```python
from build123d import *

# Parameters (mm, degrees)
SKETCH_1_W             = 60
SKETCH_1_H             = 30
EXTRUDE_1_DEPTH        = 8
CUT_EXTRUDE_1_REACH    = 10
SKETCH_2_R             = 1.2
HOLE_WIZARD_M3_1_D     = 2.5
HOLE_WIZARD_M3_1_DEPTH = 8.5
HOLE_WIZARD_M3_1_TIP   = 0.751075774
HOLE_WIZARD_M3_2_D     = 2.5
HOLE_WIZARD_M3_2_DEPTH = 8.5
HOLE_WIZARD_M3_2_TIP   = 0.751075774


with BuildPart() as part:
    # 스케치1 → 보스-돌출1 (new body)
    with BuildSketch(Plane(origin=(0, 0, 0), x_dir=(1, 0, 0), z_dir=(0, 1, 0))):
        Rectangle(SKETCH_1_W, SKETCH_1_H)
    extrude(amount=EXTRUDE_1_DEPTH)

    # 스케치2 → 컷-돌출1 (cut, up to next)
    with BuildSketch(Plane(origin=(0, 8, 0), x_dir=(1, 0, 0), z_dir=(0, 1, 0)), mode=Mode.PRIVATE) as cut_extrude_1_sk1:
        with Locations((-10, 8)):
            Circle(SKETCH_2_R)
    cut_extrude_1_tool1 = extrude(cut_extrude_1_sk1.sketch, amount=-CUT_EXTRUDE_1_REACH, mode=Mode.PRIVATE) & part.part
    add(cut_extrude_1_tool1.solids().sort_by_distance((-10, 8, -8))[0], mode=Mode.SUBTRACT)
    # 스케치2 → 컷-돌출1 (cut, up to next)
    with BuildSketch(Plane(origin=(0, 8, 0), x_dir=(1, 0, 0), z_dir=(0, 1, 0)), mode=Mode.PRIVATE) as cut_extrude_1_sk2:
        with Locations((10, 8)):
            Circle(SKETCH_2_R)
    cut_extrude_1_tool2 = extrude(cut_extrude_1_sk2.sketch, amount=-CUT_EXTRUDE_1_REACH, mode=Mode.PRIVATE) & part.part
    add(cut_extrude_1_tool2.solids().sort_by_distance((10, 8, -8))[0], mode=Mode.SUBTRACT)
    # 스케치2 → 컷-돌출1 (cut, up to next)
    with BuildSketch(Plane(origin=(0, 8, 0), x_dir=(1, 0, 0), z_dir=(0, 1, 0)), mode=Mode.PRIVATE) as cut_extrude_1_sk3:
        with Locations((10, -8)):
            Circle(SKETCH_2_R)
    cut_extrude_1_tool3 = extrude(cut_extrude_1_sk3.sketch, amount=-CUT_EXTRUDE_1_REACH, mode=Mode.PRIVATE) & part.part
    add(cut_extrude_1_tool3.solids().sort_by_distance((10, 8, 8))[0], mode=Mode.SUBTRACT)
    # 스케치2 → 컷-돌출1 (cut, up to next)
    with BuildSketch(Plane(origin=(0, 8, 0), x_dir=(1, 0, 0), z_dir=(0, 1, 0)), mode=Mode.PRIVATE) as cut_extrude_1_sk4:
        with Locations((-10, -8)):
            Circle(SKETCH_2_R)
    cut_extrude_1_tool4 = extrude(cut_extrude_1_sk4.sketch, amount=-CUT_EXTRUDE_1_REACH, mode=Mode.PRIVATE) & part.part
    add(cut_extrude_1_tool4.solids().sort_by_distance((-10, 8, 8))[0], mode=Mode.SUBTRACT)

    # M3 나사 구멍1
    with Locations(Plane.ZY.offset(30)):
        with Locations((-8, 4), (0, 4), (8, 4)):
            Hole(HOLE_WIZARD_M3_1_D / 2, depth=HOLE_WIZARD_M3_1_DEPTH)
            with Locations((0, 0, -(HOLE_WIZARD_M3_1_DEPTH + HOLE_WIZARD_M3_1_TIP / 2))):  # 118° drill point
                Cone(0, HOLE_WIZARD_M3_1_D / 2, HOLE_WIZARD_M3_1_TIP, mode=Mode.SUBTRACT)

    # M3 나사 구멍2
    with Locations(Plane(origin=(30, 0, 0), x_dir=(0, 0, -1), z_dir=(1, 0, 0))):
        with Locations((-8, 4), (0, 4), (8, 4)):
            Hole(HOLE_WIZARD_M3_2_D / 2, depth=HOLE_WIZARD_M3_2_DEPTH)
            with Locations((0, 0, -(HOLE_WIZARD_M3_2_DEPTH + HOLE_WIZARD_M3_2_TIP / 2))):  # 118° drill point
                Cone(0, HOLE_WIZARD_M3_2_D / 2, HOLE_WIZARD_M3_2_TIP, mode=Mode.SUBTRACT)


solid = part.part
```
Can you work these out from the model? Positions are in its coordinate system, mm. A direction names the side the tool comes from. Round coordinates to 2 decimals unless told otherwise and drop trailing zeros. Loops run counter-clockwise (first coordinate to the right, second up) from the corner with the lowest first, then second, coordinate; pieces in that order, holes last. Notation, with made-up numbers: M 29.25,28 L 75.25,28 A32 ccw 75.25,62 Z; hole C -8.5,-31 d1. An arc over 180 degrees is marked long. Answer in a Markdown table with one row per item.
1. Please list where these lines run through material, in increasing order: line 1 (Z direction, x = 27.25, y = 4); line 2 (Z direction, x = -10, y = 2); line 3 (X direction, y = 1.75, z = 8). Write a range as from..to.
Established:
| item | result |
|---|---|
| line 1 | -15..-9.25, -6.75..-1.25, 1.25..6.75, 9.25..15 |
| line 2 | -15..-9.2, -6.8..6.8, 9.2..15 |
| line 3 | -30..-11.2, -8.8..8.8, 11.2..30 |
2. Thinking about a two-plate mould opening in X: for faces 4 (the face through (25.69, 2.78, -0.27)), 5 (the face through (30, 6, 0)), 6 (the face through (-8.855, 4.056, -8.36)), which applies, pulls with the +X half, pulls with the -X half, needs draft (parallel to the pull), parting line crosses it, or undercut?
Established:
| item | result |
|---|---|
| face 4 | needs draft |
| face 5 | pulls with the +X half |
| face 6 | undercut |
3. If we section it at A-A, the plane x = 10: Please give me the cut outline in (y, z), plus the area to 3 significant figures.
Established:
| item | result |
|---|---|
| outline | M 0,-15 L 8,-15 L 8,-9.2 L 0,-9.2 Z; M 0,-6.8 L 8,-6.8 L 8,6.8 L 0,6.8 Z; M 0,9.2 L 8,9.2 L 8,15 L 0,15 Z |
| area | 202 mm² |
4. I'm going to push flat-ended pins straight in: pin 1 Ø1.5 at (y, z) = (4, -8) entering from +X; pin 2 Ø2 at (y, z) = (4, -8) entering from +X. Where does each tip first touch, or does it pass through?
Established:
| item | result |
|---|---|
| pin 1 | x = 21.2 |
| pin 2 | x = 21.35 |
5. On a 3-axis mill with a long thin cutter (end or side, diameter ignored), from which of +Z, -Z, +X, -X, +Y, -Y can I reach the whole of each face in a straight line? I mean faces 1 (the face through (9.116, 4.056, -8.811)), 2 (the face through (25.69, 3.24, 7.01)), 3 (the face through (-25.69, 3.24, -7.01)). Say none if no direction works.
Established:
| item | result |
|---|---|
| face 1 | +Y, -Y |
| face 2 | +X |
| face 3 | -X |
